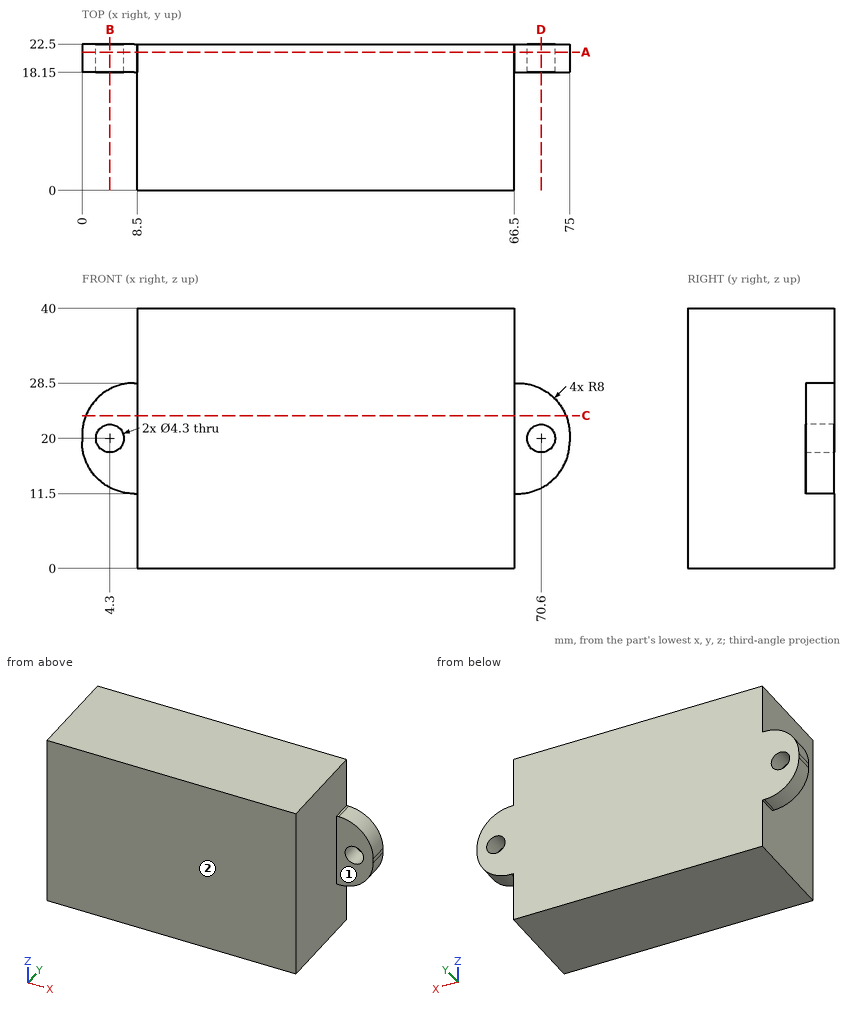
Design review of the part shown in the three views and the two pictorial views. Dimensions are in mm from the part's minimum x, y and z. A direction names the side the tool comes from. Coordinates: 2 decimals unless noted, no trailing zeros. Loops run counter-clockwise (first coordinate to the right, second up) from the corner with the lowest first, then second, coordinate; pieces in that order, holes last. Notation, with made-up numbers: M 57.25,42 L 110.25,42 A13 ccw 110.25,54 Z; hole C 73,73 d10. An arc over 180 degrees is marked long. Put each result on its own line as item: value. Start each with the question number.
Q1. Wall thickness on line 1 (X direction, y = 19.8, z = 20); line 2 (Y direction, x = 6.5, z = 20); line 3 (X direction, y = 9.5, z = 7): over which ranges is each line inside the solid? List them lowest first.
Q2. Add section B-B (x = 4.3). Write out the cut boundary in (y, z).
Q3. Add section D-D (x = 70.6). Write out the cut boundary in (y, z), and give its area (3 significant figures).
Q4. Add section C-C (z = 23.5). Write out the cut boundary in (x, y), and give its area (3 significant figures).
Q5. Add section A-A (y = 21.25). Write out the cut boundary in (x, z), and give its area (3 significant figures).
Q6. For the marked faces 1 and 2, list the 3-axis set-ups (+Z, -Z, +X, -X, +Y, -Y) from which the entire face can be reached by the end or side of a thin tool; tool diameter is ignored.
Q7. Clearance check with flat-ended pins moving along their axes: pin 1 (1.5 mm diameter, centred on y = 14.5, z = 4.5, fed in from -X); pin 2 (1 mm diameter, centred on y = 18.5, z = 5, fed in from +X); pin 3 (4 mm diameter, centred on x = 69, z = 20, fed in from -Y). State where each tip first meets the part, or that it passes through.
Answers:
1. line 1: x = 0 to 2.15, 6.45 to 68.45, 72.75 to 75
1. line 2: y = 18.15 to 22.5
1. line 3: x = 8.5 to 66.5
2. outline: M 18.15,12.41 L 22.5,12.41 L 22.5,17.85 L 18.15,17.85 Z; M 18.15,22.15 L 22.5,22.15 L 22.5,27.59 L 18.15,27.59 Z
3. outline: M 18.15,12.36 L 22.5,12.36 L 22.5,17.85 L 18.15,17.85 Z; M 18.15,22.15 L 22.5,22.15 L 22.5,27.64 L 18.15,27.64 Z
3. area: 47.8 mm^2
4. outline: M 0.58,18.15 L 8.5,18.15 L 8.5,0 L 66.5,0 L 66.5,18.15 L 74.42,18.15 L 74.42,22.5 L 0.58,22.5 Z
4. area: 1,370 mm^2
5. outline: M 0,19.5 A8 ccw 8,11.5 L 8.5,11.5 L 8.5,0 L 66.5,0 L 66.5,11.5 L 67,11.5 A8 ccw 75,19.5 L 75,20.5 A8 ccw 67,28.5 L 66.5,28.5 L 66.5,40 L 8.5,40 L 8.5,28.5 L 8,28.5 A8 ccw 0,20.5 Z; hole C 4.3,20 d4.3; hole C 70.6,20 d4.3
5. area: 2,530 mm^2
6. face 1: +Z, -Z, +X, -Y
6. face 2: +Z, -Z, +X, -X, -Y
7. pin 1: stops at x = 8.5
7. pin 2: stops at x = 66.5
7. pin 3: stops at y = 18.15
